Here's how the part is built. I have some questions about the finished solid (model axes, mm). A direction names the side the tool comes from. Round coordinates to 2 decimals unless told otherwise and drop trailing zeros. Write each loop counter-clockwise with the first axis right and the second up, starting at its lowest first coordinate (ties: lowest second). Pieces come first, ordered by that corner, then holes. Notation, with made-up numbers: (48.5, 73) -> (96.5, 73) arc R18 ccw to (96.5, 102) -> close; hole circle Ø8 at (-2.75, 41.25). An arc over 180 degrees is marked (long way). Put each result on its own line as item: value. Start each with the question number.
1. Suppose I cut it at A-A (y = -73.5). Please give me the cut outline in (x, z), then the cut area to 3 significant figures.
2. I need wall thicknesses on probe 1 along X at (y, z) = (-93.5, 26); probe 2 along Y at (x, z) = (6, 14.5). Which ranges of each line are inside material? Lowest first, please. Write a range as from..to.
3. For pin 1 (3.5 mm diameter, centred on x = 98.5, y = -41.5, fed in from +Z), with a flat end and sliding along its axis, tell me the tip position at first contact or that it passes through.
4. Suppose I cut it at B-B (z = 32). Please give me the cut outline in (x, y), then the cut area to 3 significant figures.
5. Suppose I cut it at C-C (x = 77.5). Please give me the cut outline in (y, z).
6. We'd pull the mould along Y, two halves only. Please class faces 1 (the face through (49, 0, 25)), 2 (the face through (98, -50, 47)), 3 (the face through (75, -99, 48)), 4 (the face through (98, -75, 48)): +Y half, -Y half, draft (parallel to the pull), parting line (faces both ways), or undercut.
7. Which directions (+Z, -Z, +X, -X, +Y, -Y) give clear straight access to the entire face, cutting with the end or side of a thin tool? Please do faces 5 (the face through (1, -25, 48)), 6 (the face through (49, -97, 25)), 7 (the face through (50, -2, 47)).
```python
from build123d import *

# Parameters (mm, degrees)
SKETCH_1_W          = 100
SKETCH_1_H          = 100
SKETCH_1_W_2        = 94
SKETCH_1_H_2        = 94
EXTRUDE_1_DEPTH     = 50
SKETCH_2_W          = 3
SKETCH_2_H          = 50
CUT_EXTRUDE_1_DEPTH = 151
SKETCH_3_W          = 50
SKETCH_3_H          = 3
CUT_EXTRUDE_2_DEPTH = 151


with BuildPart() as part:
    # 草图1 → 凸台-拉伸1 (new body)
    with BuildSketch(Plane.XY):
        with Locations((50, -50)):
            Rectangle(SKETCH_1_W, SKETCH_1_H)
        with Locations((50, -50)):
            Rectangle(SKETCH_1_W_2, SKETCH_1_H_2, mode=Mode.SUBTRACT)
    extrude(amount=EXTRUDE_1_DEPTH)

    # 草图2 → 切除-拉伸1 (cut, through all)
    with BuildSketch(Plane.ZY):
        with Locations((48.5, -50)):
            Rectangle(SKETCH_2_W, SKETCH_2_H)
    extrude(amount=-CUT_EXTRUDE_1_DEPTH, mode=Mode.SUBTRACT)

    # 草图3 → 切除-拉伸2 (cut, through all)
    with BuildSketch(Plane.XZ.offset(100)):
        with Locations((50, 48.5)):
            Rectangle(SKETCH_3_W, SKETCH_3_H)
    extrude(amount=-CUT_EXTRUDE_2_DEPTH, mode=Mode.SUBTRACT)


solid = part.part
```
Verdict:
1. outline: (0, 0) -> (3, 0) -> (3, 47) -> (0, 47) -> close; (97, 0) -> (100, 0) -> (100, 47) -> (97, 47) -> close
1. area: 282 mm^2
2. probe 1: x = 0..3, 97..100
2. probe 2: y = -100..-97, -3..0
3. pin 1: stops at z = 47
4. outline: (0, -100) -> (100, -100) -> (100, 0) -> (0, 0) -> close; hole (3, -97) -> (97, -97) -> (97, -3) -> (3, -3) -> close
4. area: 1,160 mm^2
5. outline: (-100, 0) -> (-97, 0) -> (-97, 50) -> (-100, 50) -> close; (-3, 0) -> (0, 0) -> (0, 50) -> (-3, 50) -> close
6. face 1: +Y half
6. face 2: undercut
6. face 3: draft
6. face 4: undercut
7. face 5: +Z, +X, -X
7. face 6: +Z, -Z
7. face 7: +Z, +Y, -Y
